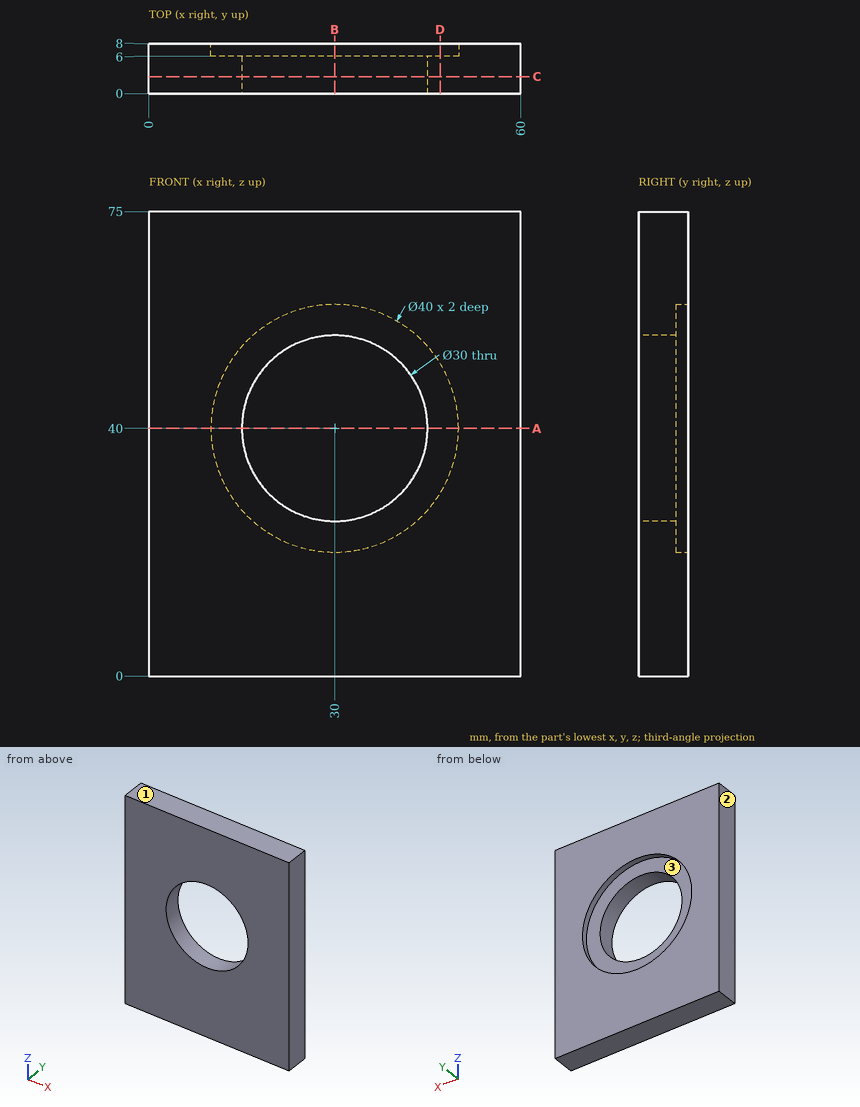
Verification items for this drawing (mm, ordinates from the low corner). Coordinates: 2 decimals unless noted, no trailing zeros. Loops run counter-clockwise (first coordinate to the right, second up) from the corner with the lowest first, then second, coordinate; pieces in that order, holes last.
Item 1: Sectioned sample at A-A, the plane z = 40. Record the boundary of the cut face in (x, y).
Item 2: Sectioned sample at D-D, the plane x = 47. Record the boundary of the cut face in (y, z).
Item 3: Sectioned sample at C-C, the plane y = 2.75. Record the boundary of the cut face in (x, z), then the cut area to 3 significant figures.
Item 4: Thickness scan on line 1 (Z direction, x = 29.5, y = 7.75); line 2 (X direction, y = 6.5, z = 25); line 3 (Z direction, x = 42.5, y = 6.75). Record the ranges inside material, lowest first.
Item 5: Release check for a two-part mould opening along X. For the marked faces 1, 2 and 3 record: released by +X, released by -X, zero draft, split by the parting line, or undercut.
Item 6: Go/stop test with a flat-tipped pin: pin 1 Ø3 at (x, y) = (42, 3.5) entering from -Z. Record where the tip stops, or that it passes through.
Item 7: Sectioned sample at B-B, the plane x = 30. Record the boundary of the cut face in (y, z).
Check result:
1. outline: (0, 0) - (15, 0) - (15, 6) - (10, 6) - (10, 8) - (0, 8) - close; (45, 0) - (60, 0) - (60, 8) - (50, 8) - (50, 6) - (45, 6) - close
2. outline: (0, 0) - (8, 0) - (8, 29.46) - (6, 29.46) - (6, 50.54) - (8, 50.54) - (8, 75) - (0, 75) - close
3. outline: (0, 0) - (60, 0) - (60, 75) - (0, 75) - close; hole circle Ø30 at (30, 40)
3. area: 3,790 mm2
4. line 1: z = 0 to 20.01, 59.99 to 75
4. line 2: x = 0 to 16.77, 43.23 to 60
4. line 3: z = 0 to 24.39, 55.61 to 75
5. face 1: zero draft
5. face 2: released by -X
5. face 3: undercut
6. pin 1: stops at z = 0
7. outline: (0, 0) - (8, 0) - (8, 20) - (6, 20) - (6, 25) - (0, 25) - close; (0, 55) - (6, 55) - (6, 60) - (8, 60) - (8, 75) - (0, 75) - close
